Autodesk Inventor part; units mm, degrees
ref_plane "YZ Plane" through (0, 0, 0) normal (1, 0, 0) x (0, 1, 0)
ref_plane "XZ Plane" through (0, 0, 0) normal (0, 1, 0) x (-1, 0, 0)
ref_plane "XY Plane" through (0, 0, 0) normal (0, 0, 1) x (1, 0, 0)
sketch "Sketch2" plane through (0, 0, 0) normal (0, 0, 1) x (1, 0, 0)
  line L0 (0, 0) -> (40, 0) construction
  line L1 (40, 0) -> (40, -40) construction
  line L2 (40, -40) -> (0, -40) construction
  line L3 (0, -40) -> (0, 0) construction
  line L4 (43, 0) -> (43, -43)
  line L5 (43, -43) -> (0, -43)
  line L6 (0, -43) -> (0, -102.2254)
  line L7 (0, -102.2254) -> (40, -102.2254)
  line L8 (40, -102.2254) -> (102.2254, -40)
  line L9 (102.2254, -40) -> (102.2254, 0)
  line L10 (102.2254, 0) -> (43, 0)
  line L11 (43, -43) -> (71.1127, -71.1127) construction
  circle A0 centre (61.2132, -61.2132) radius 7
  dimension "d7" = 40
  dimension "d8" = 40
  dimension "d9" = 3
  dimension "d10" = 3
  dimension "d11" = 14
  dimension "d12" = 30
  dimension "d13" = 14
extrude "Plate2" add sketch "Sketch2" along normal blind 3
fillet "Corner Round3" radius 3 7 edges at (0, -102.2254, 1.5) (0, -43, 1.5) (43, -43, 1.5) (43, 0, 1.5) (102.2254, 0, 1.5) (102.2254, -40, 1.5) (40, -102.2254, 1.5)
feature "Corner Round4" [suppressed]
sketch "Sketch3" plane through (43, -103.468, 3) normal (-0.7071068, 0.7071068, 0) x (-0.7071068, -0.7071068, 0)
  line L0 (-85.5147, 0) -> (0, 0)
  line L1 (0, 0) -> (0, -20)
  line L2 (0, -20) -> (-85.5147, -20)
  line L3 (-85.5147, -20) -> (-85.5147, 0)
equation "\"d8\" = d7"
equation "\"d10\" = d9"
equation "\"d13\" = d11"
equation "\"d14\" = Thickness"
equation "\"BendReliefWidth\" = Thickness"
equation "\"BendReliefDepth\" = 0.5 * Thickness"
equation "\"CornerReliefSize\" = 4 * Thickness"
equation "\"MinimumRemnant\" = 2 * Thickness"
equation "\"TransitionRadius\" = BendRadius"
equation "\"JacobiRadiusSize\" = BendRadius"
equation "\"GapSize\" = Thickness"
properties part number "GNH 081 leg support" material "Stainless Steel"
Work out the finished part from the listing and answer in its coordinate system (mm). A direction names the side the tool comes from. Give positions to 0.01 mm unless a question says otherwise; leave off trailing zeros. Order: outer loops, then holes, each group sorted by start corner. A loop starts at its lowest first (then second) coordinate and runs counter-clockwise, first axis right, second up. Notation, with made-up numbers: (69.5, 80.25) - (125.5, 80.25) arc R16 ccw to (125.5, 93.25) - close; hole circle Ø2 at (29, 17.25). An arc over 180 degrees is marked (long way). Answer as CSV lines item,"result". Start each with the question number.
Q1. Given pin 1 Ø1.5 at (x, z) = (15.5, 1.5) entering from +Y, flat-ended and moving along its own axis, determine where the tip first touches the part or whether it passes through.
Q2. The part is cut by section B-B (x = 11). Write down the section's boundary in (y, z).
Q3. The mould has two halves that part along Y. Classify faces 3 (the face through (0, -72, 1)), 4 (the face through (67.89, -63.32, 1.48)), 5 (the face through (0.9, -43.86, 1.52)): +Y half, -Y half, draft (parallel to the pull), parting line (faces both ways), or undercut.
Q4. The part is cut by section C-C (y = -34.5). Write down the section's boundary in (x, z).
Q5. Find the intervals of material crossed by L1, parallel to X at y = -16.5, z = 1.05; L2, parallel to Y at x = 18, z = 1.8; L3, parallel to Y at x = 88, z = 1.3, in increasing order. Write a range as [from, to].
Q6. For faces 1 (the face through (43, -21, 1)), 2 (the face through (101.37, -0.9, 1.52)), determine the directions among +Z, -Z, +X, -X, +Y, -Y from which every point of the face is accessible in a straight line to the end or side of a thin tool.
Q7. The part is cut by section A-A (z = 0.55). Write down the section's boundary in (x, y), then the cut area to 3 significant figures.
Check result:
1,pin 1,"stops at y = -43"
2,outline,"(-102.23, 0) - (-43, 0) - (-43, 3) - (-102.23, 3) - close"
3,face 3,"draft"
3,face 4,"undercut"
3,face 5,"+Y half"
4,outline,"(43, 0) - (102.23, 0) - (102.23, 3) - (43, 3) - close"
5,L1,"x = [43, 102.23]"
5,L2,"y = [-102.23, -43]"
5,L3,"y = [-54.23, 0]"
6,face 1,"+Z, -Z, -X, +Y"
6,face 2,"+Z, -Z, +X, +Y"
7,outline,"(0, -99.23) arc R3 ccw to (3, -102.23) - (38.76, -102.23) arc R3 ccw to (40.88, -101.35) - (101.35, -40.88) arc R3 ccw to (102.23, -38.76) - (102.23, -3) arc R3 ccw to (99.23, 0) - (46, 0) arc R3 ccw to (43, -3) - (43, -40) arc R3 cw to (40, -43) - (3, -43) arc R3 ccw to (0, -46) - close; hole circle Ø14 at (61.21, -61.21)"
7,area,"6,500 mm²"
